Part print with two shaded views. Sizes in mm from the minimum x, y, z corner. Round coordinates to 2 decimals unless told otherwise and drop trailing zeros. Write each loop counter-clockwise with the first axis right and the second up, starting at its lowest first coordinate (ties: lowest second). Pieces come first, ordered by that corner, then holes. Notation, with made-up numbers: M 14,23 L 66,23 A15 cw 66,36 Z; hole C -35.75,16.25 d5. An arc over 180 degrees is marked long. Use one line per item in the form item = value. Start each with the question number.
Item 1: Cut at A-A, the plane x = 5. Give the cut face in (y, z), then the cut area to 3 significant figures.
Item 2: Probe L1, parallel to Z at x = 30, y = 2.3; L2, parallel to X at y = 1.8, z = 36. List the from-to ranges inside material, lowest first.
Item 3: Cut at B-B, the plane z = 36. Give the cut face in (x, y).
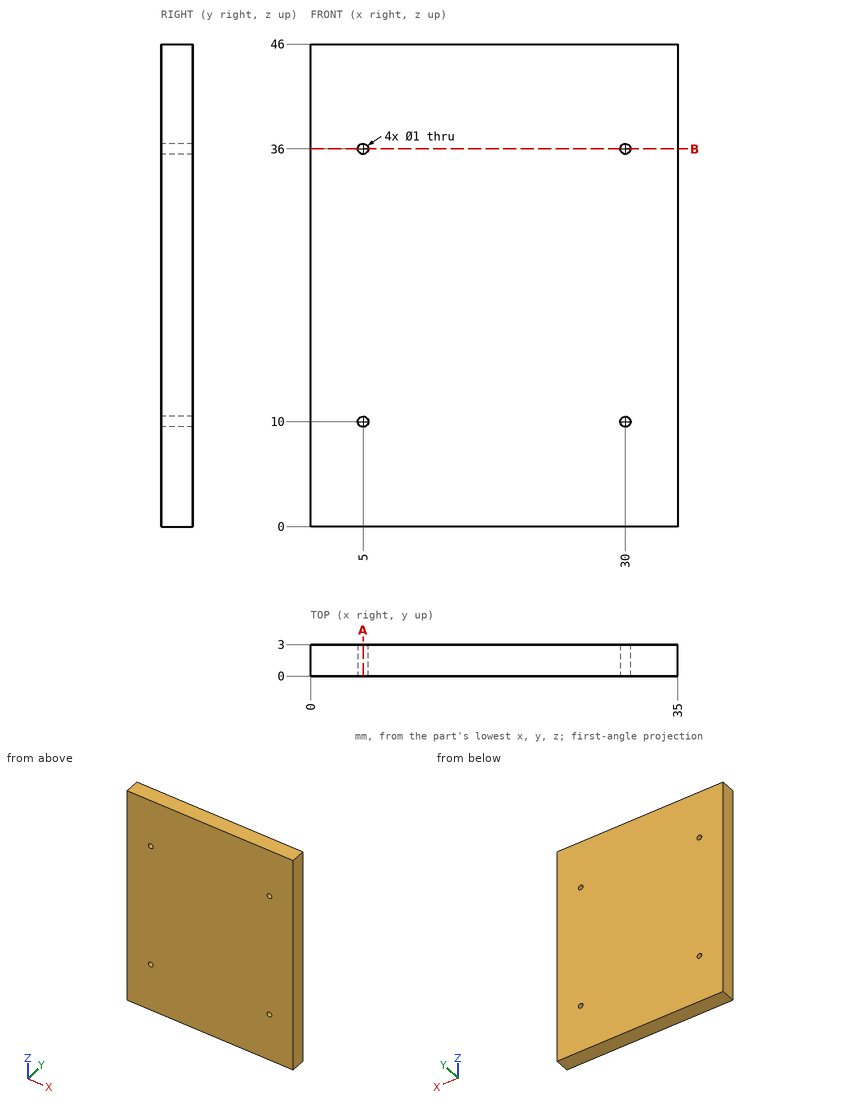
Model answer:
q1.outline = M 0,0 L 3,0 L 3,9.5 L 0,9.5 Z; M 0,10.5 L 3,10.5 L 3,35.5 L 0,35.5 Z; M 0,36.5 L 3,36.5 L 3,46 L 0,46 Z
q1.area = 132 mm²
q2.L1 = 0 to 9.5, 10.5 to 35.5, 36.5 to 46
q2.L2 = 0 to 4.5, 5.5 to 29.5, 30.5 to 35
q3.outline = M 0,0 L 4.5,0 L 4.5,3 L 0,3 Z; M 5.5,0 L 29.5,0 L 29.5,3 L 5.5,3 Z; M 30.5,0 L 35,0 L 35,3 L 30.5,3 Z
